The listing builds one solid part. Answer for the finished solid, in the listing's coordinates (mm). Face numbers are marked on the shaded views. A direction names the side the tool comes from. Coordinates: 2 decimals unless noted, no trailing zeros. Write each loop counter-clockwise with the first axis right and the second up, starting at its lowest first coordinate (ties: lowest second). Pieces come first, ordered by that corner, then holes. Notation, with made-up numbers: M -40,82.25 L -20,82.25 A17 ccw -20,99.25 Z; hole C 38,-3.5 d3. An arc over 180 degrees is marked long. Answer as a JSON object with one key per item and string values. Group by question number.
from build123d import *

# Parameters (mm, degrees)
SKETCH1_W           = 5.5
SKETCH1_H           = 5.5
BOSS_EXTRUDE1_DEPTH = 1.2
SKETCH2_R           = 2.1
BOSS_EXTRUDE2_DEPTH = 2
SKETCH3_R           = 1.95
CUT_EXTRUDE1_DEPTH  = 0.9
CHAMFER2_SIZE       = 0.3
CHAMFER2_SIZE2      = 1.119615242


with BuildPart() as part:
    # Sketch1 → Boss-Extrude1 (new body)
    with BuildSketch(Plane(origin=(0, 0, 0), x_dir=(1, 0, 0), z_dir=(0, 1, 0))):
        Rectangle(SKETCH1_W, SKETCH1_H)
    extrude(amount=BOSS_EXTRUDE1_DEPTH)

    # Sketch2 → Boss-Extrude2 (add)
    with BuildSketch(Plane(origin=(0, 1.2, 0), x_dir=(1, 0, 0), z_dir=(0, 1, 0))):
        with Locations(Location((0, 0, 0), (0, 0, 270))):
            Circle(SKETCH2_R)
    extrude(amount=BOSS_EXTRUDE2_DEPTH)

    # Sketch3 → Cut-Extrude1 (cut)
    with BuildSketch(Plane.XZ):
        with Locations(Location((0, 0, 0), (0, 0, 270))):
            Circle(SKETCH3_R)
    extrude(amount=-CUT_EXTRUDE1_DEPTH, mode=Mode.SUBTRACT)

    # Chamfer2
    chamfer2_edges = [part.edges().sort_by_distance(p)[0] for p in [
        (0, 3.2, -2.1),
    ]]
    chamfer2_side = [part.faces().sort_by_distance(p)[0] for p in [
        (0, 3.2, 0),
    ]]
    chamfer(chamfer2_edges, length=CHAMFER2_SIZE, length2=CHAMFER2_SIZE2, reference=chamfer2_side[0])


solid = part.part
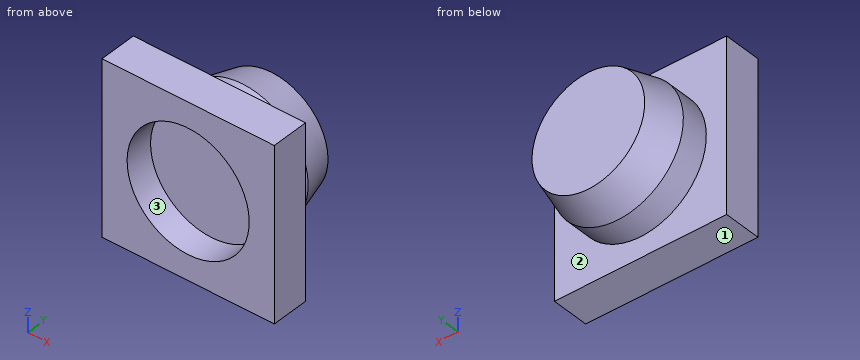
Item 1: A cutting plane is placed at B-B, the plane x = 0. Write down the section's boundary in (y, z).
Item 2: A cutting plane is placed at D-D, the plane y = 1.8. Write down the section's boundary in (x, z), and give its area (3 significant figures).
Item 3: A cutting plane is placed at A-A, the plane y = 0.5. Write down the section's boundary in (x, z), and give its area (3 significant figures).
Item 4: A cutting plane is placed at C-C, the plane z = 0. Write down the section's boundary in (x, y), and give its area (3 significant figures).
Item 5: Consider L1, parallel to X at y = 0.55, z = 0; L2, parallel to Y at x = -0.7, z = -1.05; L3, parallel to Y at x = 1.15, z = -2.15. Determine where each line is inside the solid, lowest interval first. Write a range as from..to.
Item 6: A tool of negligible diameter and unlimited length cuts with its end or side. For the marked faces 1, 2 and 3, from which of +Z, -Z, +X, -X, +Y, -Y can it reach the whole face along a straight path? Write none if from no direction.
Answer:
{
 "1": {"outline": "M 0,-2.75 L 1.2,-2.75 L 1.2,-2.1 L 2.08,-2.1 L 3.2,-1.8 L 3.2,1.8 L 2.08,2.1 L 1.2,2.1 L 1.2,2.75 L 0,2.75 L 0,1.95 L 0.9,1.95 L 0.9,-1.95 L 0,-1.95 Z"},
 "2": {"outline": "C 0,0 d4.2", "area": "13.9 mm2"},
 "3": {"outline": "M -2.75,-2.75 L 2.75,-2.75 L 2.75,2.75 L -2.75,2.75 Z; hole C 0,0 d3.9", "area": "18.3 mm2"},
 "4": {"outline": "M -2.75,0 L -1.95,0 L -1.95,0.9 L 1.95,0.9 L 1.95,0 L 2.75,0 L 2.75,1.2 L 2.1,1.2 L 2.1,2.08 L 1.8,3.2 L -1.8,3.2 L -2.1,2.08 L -2.1,1.2 L -2.75,1.2 Z", "area": "11.2 mm2"},
 "5": {"L1": "-2.75..-1.95, 1.95..2.75", "L2": "0.9..3.2", "L3": "0..1.2"},
 "6": {"face 1": "-Z, +X, -X, +Y, -Y", "face 2": "+Y", "face 3": "-Y"}
}
